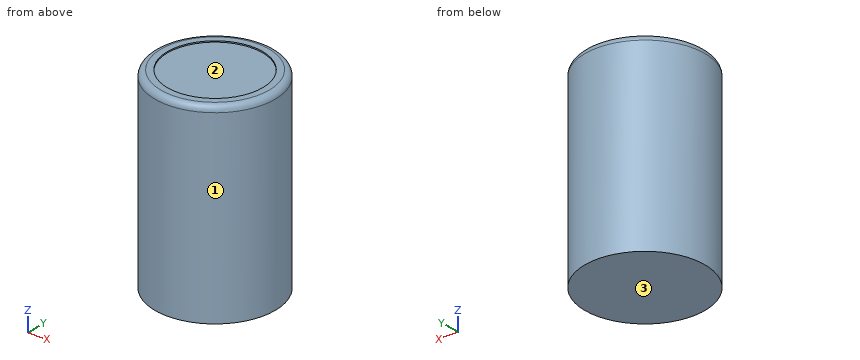
Autodesk Inventor part; units mm, degrees
ref_plane "YZ Plane" through (0, 0, 0) normal (1, 0, 0) x (0, 1, 0)
ref_plane "XZ Plane" through (0, 0, 0) normal (0, 1, 0) x (-1, 0, 0)
ref_plane "XY Plane" through (0, 0, 0) normal (0, 0, 1) x (1, 0, 0)
sketch "Sketch1" plane through (0, 0, 0) normal (0, 0, 1) x (1, 0, 0)
  circle A0 centre (0, 0) radius 6.35
  dimension "d0" = 12.7
extrude "Extrusion1" add sketch "Sketch1" along normal mid plane 20.32
fillet "Fillet1" radius 0.635 1 edges at (-6.35, 0, 10.16)
sketch "Sketch2" plane through (0, 0, 10.16) normal (0, 0, 1) x (1, 0, 0)
  circle A0 centre (0, 0) radius 5.715
  circle A1 centre (0, 0) radius 5.0354
extrude "Extrusion2" cut sketch "Sketch2" against normal blind 0.127 contours A1
properties part number "Capacitor"
Geometry: final body of the model. Coordinates: model frame, mm. Face numbers are marked on the shaded views. Round coordinates to 2 decimals unless told otherwise and drop trailing zeros. Order: outer loops, then holes, each group sorted by start corner. A loop starts at its lowest first (then second) coordinate and runs counter-clockwise, first axis right, second up. Notation, with made-up numbers: M 85,52.5 L 130,52.5 A34 ccw 130,90.5 Z; hole C -11.5,39 d4. An arc over 180 degrees is marked long. Use one line per item in the form item = value. Start each with the question number.
Q1. Cut plane A-A (z = 4.5). Return loops of the section in (x, y).
Q2. Pin query (flat end, axial travel): pin 1 Ø1 at (y, z) = (3.5, -3) entering from +X; pin 2 Ø1.5 at (x, z) = (2.5, 1) entering from -Y; pin 3 Ø3 at (x, z) = (-2.5, -3.5) entering from -Y. Return the tip coordinate at first contact, or that it passes through.
Q3. Material intervals for line 1 (Z direction, x = 0.75, y = -3.25); line 2 (Y direction, x = 3.75, z = 3); line 3 (X direction, y = -4, z = 0.5), sorted ascending. Write a range as [from, to].
Q4. Mould query, pull axis Y, two halves, no side actions, for the marked faces 1, 2 and 3. Classes: +Y half, -Y half, draft (parallel to the pull), parting line (faces both ways), or undercut.
Geometry results:
q1.outline = C 0,0 d12.7
q2.pin_1 = 5.6
q2.pin_2 = -6.1
q2.pin_3 = -6.27
q3.line_1 = [-10.16, 10.03]
q3.line_2 = [-5.12, 5.12]
q3.line_3 = [-4.93, 4.93]
q4.face_1 = parting line
q4.face_2 = undercut
q4.face_3 = draft
